Source: CAD feature listing. Evaluate the final solid. Frame: model axes, mm. Face numbers are marked on the shaded views. A direction names the side the tool comes from. Give positions to 0.01 mm unless a question says otherwise; leave off trailing zeros. Order: outer loops, then holes, each group sorted by start corner. A loop starts at its lowest first (then second) coordinate and runs counter-clockwise, first axis right, second up. Notation, with made-up numbers: M 76.25,8 L 133.25,8 A22 cw 133.25,38 Z; hole C 1,40.5 d8. An arc over 180 degrees is marked long. Answer as a JSON object with one key per item and string values. Group by question number.
1. Pin query (flat end, axial travel): P1, Ø6, axis at x = 14, y = 11.5, coming from the +Z side (3 decimals); P2, Ø1.3, axis at x = -0.5, z = -34, coming from the -Y side; P3, Ø1.3, axis at x = -0.5, y = 1.5, coming from the +Z side (3 decimals); P4, Ø4.5, axis at y = 4.15, z = -61.79, coming from the -X side (1 decimal). Return the tip coordinate at first contact, or that it passes through.
2. Set-up query: the marked faces 4 and 5. Return all of +Z, -Z, +X, -X, +Y, -Y with unobstructed straight access to the full face (end or side cutting, diameter ignored); none if empty.
3. Material intervals for L1, parallel to X at y = 5, z = -16.5 (1 decimal); L2, parallel to Y at x = 8.5, z = -21.5 (1 decimal); L3, parallel to Y at x = 16.25, z = -6, sorted ascending. Write a range as [from, to].
4. Pull-direction query (X, two-part tool) for the marked faces 1, 2 and 3; classes: +X half, -X half, draft (parallel to the pull), parting line (faces both ways), or undercut.
5. Section query B-B (z = -60.5). Output: boundary loops of the cut face in (x, y) (1 decimal), plus the area to 3 significant figures.
6. Section query D-D (z = -19). Output: boundary loops of the cut face in (x, y) (1 decimal), plus the area to 3 significant figures.
7. Section query C-C (y = 5). Count the separate pieces of the cut face and the enclosed holes in it, plus the area to 3 significant figures.
8. Section query A-A (y = 10.75). Output: boundary loops of the cut face in (x, z) (1 decimal), plus the area to 3 significant figures.
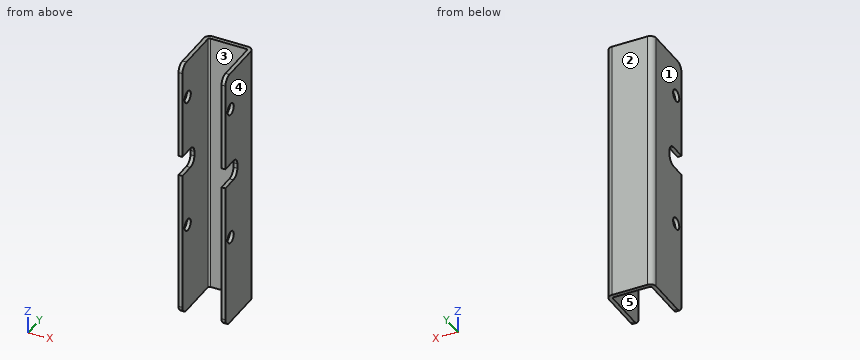
from build123d import *

# Parameters (mm, degrees)
BASE_FLANGE1_DEPTH           = 1.5875
EDGE_FLANGE1_STRIP_W         = 7.8232
EDGE_FLANGE1_STRIP_H         = 1.5875
EDGE_FLANGE1_STRIP_CUT_DEPTH = 107.95
EDGE_FLANGE1_DEPTH           = 107.95
EDGE_FLANGE2_STRIP_W         = 7.8232
EDGE_FLANGE2_STRIP_H         = 1.5875
EDGE_FLANGE2_STRIP_CUT_DEPTH = 107.95
EDGE_FLANGE2_DEPTH           = 107.95
HOLE1_START                  = -1.5875
HOLE1_OUTLINE_R              = 2.413
HOLE1_DEPTH                  = 19.05
CUT_EXTRUDE1_DEPTH           = 103.402979235
CUT_EXTRUDE1_DEPTH_BACK      = 103.402979235
SKETCH27_W                   = 8.255
SKETCH27_H                   = 9.364783331
FILLET1_R                    = 3.175


# Read off the part's stored shape, not the designer's step: Hole1
# Sheet-metal steps are written as plain solids
with BuildPart() as part:
    # Sketch1 → Base-Flange1 (new body)
    with BuildSketch(Plane(origin=(0, 0, 0), x_dir=(0, 0, -1), z_dir=(1, 0, 0))):
        Polygon((0, 0), (88.9, 0), (98.425, 0), (98.425, 22.225), (88.9, 22.225), (0, 22.225), (-9.525, 22.225), (-9.525, 0), align=None)
    extrude(amount=-BASE_FLANGE1_DEPTH)

    # Edge-Flange1 strip (across the edge) → Edge-Flange1 strip cut (cut)
    with BuildSketch(Plane(origin=(0, 22.225, -98.425), x_dir=(0, -1, 0), z_dir=(0, 0, 1))):
        with Locations((-1.5875, -0.79375)):
            Rectangle(EDGE_FLANGE1_STRIP_W, EDGE_FLANGE1_STRIP_H)
    extrude(amount=EDGE_FLANGE1_STRIP_CUT_DEPTH, mode=Mode.SUBTRACT)

    # Edge-Flange1 section (across the edge) → Edge-Flange1 (add)
    with BuildSketch(Plane(origin=(0, 22.225, -98.425), x_dir=(0, -1, 0), z_dir=(0, 0, 1))):
        with BuildLine():
            Line((0, 0.7366), (0, 17.4625))
            Line((0, 17.4625), (1.5875, 17.4625))
            Line((1.5875, 17.4625), (1.5875, 0.7366))
            ThreePointArc((1.5875, 0.7366), (1.803245145, 0.215745145), (2.3241, 0))
            Line((2.3241, 0), (2.3241, -1.5875))
            ThreePointArc((2.3241, -1.5875), (0.68071313, -0.90678687), (0, 0.7366))
        make_face()
    extrude(amount=EDGE_FLANGE1_DEPTH)

    # Edge-Flange2 strip (across the edge) → Edge-Flange2 strip cut (cut)
    with BuildSketch(Plane(origin=(17.4625, 20.6375, -98.425), x_dir=(-1, 0, 0), z_dir=(0, 0, 1))):
        with Locations((-1.5875, -0.79375)):
            Rectangle(EDGE_FLANGE2_STRIP_W, EDGE_FLANGE2_STRIP_H)
    extrude(amount=EDGE_FLANGE2_STRIP_CUT_DEPTH, mode=Mode.SUBTRACT)

    # Edge-Flange2 section (across the edge) → Edge-Flange2 (add)
    with BuildSketch(Plane(origin=(17.4625, 20.6375, -98.425), x_dir=(-1, 0, 0), z_dir=(0, 0, 1))):
        with BuildLine():
            Line((0, 0.7366), (0, 20.6375))
            Line((0, 20.6375), (1.5875, 20.6375))
            Line((1.5875, 20.6375), (1.5875, 0.7366))
            ThreePointArc((1.5875, 0.7366), (1.803245145, 0.215745145), (2.3241, 0))
            Line((2.3241, 0), (2.3241, -1.5875))
            ThreePointArc((2.3241, -1.5875), (0.68071313, -0.90678687), (0, 0.7366))
        make_face()
    extrude(amount=EDGE_FLANGE2_DEPTH)

    # Hole1 outline → Hole1 (cut)
    with BuildSketch(Plane.YZ.offset(HOLE1_START)):
        with Locations((4.148353843, -61.790618702)):
            Circle(HOLE1_OUTLINE_R)
        with Locations((4.148353843, -6.164618702)):
            Circle(HOLE1_OUTLINE_R)
    extrude(amount=HOLE1_DEPTH, mode=Mode.SUBTRACT)

    # Sketch27 → Cut-Extrude1 (cut, two sides: drawn at the far end of the back side and taken through both)
    with BuildSketch(Plane(origin=(0, 0, 0), x_dir=(0, 0, -1), z_dir=(1, 0, 0)).offset(-CUT_EXTRUDE1_DEPTH_BACK)):
        with Locations((33.9725, 4.682391665)):
            Rectangle(SKETCH27_W, SKETCH27_H)
    extrude(amount=CUT_EXTRUDE1_DEPTH + CUT_EXTRUDE1_DEPTH_BACK, mode=Mode.SUBTRACT)

    # Fillet1
    fillet1_edges = [part.edges().sort_by_distance(p)[0] for p in [
        (-0.79375, 9.364783331, -29.845),
        (-0.79375, 9.364783331, -38.1),
        (16.66875, 9.364783331, -29.845),
        (16.66875, 9.364783331, -38.1),
        (-0.79375, 0, 9.525),
        (-0.79375, 0, -98.425),
        (16.66875, 0, -98.425),
        (16.66875, 0, 9.525),
    ]]
    fillet(fillet1_edges, radius=FILLET1_R)


solid = part.part
Answer sheet:
{
 "1": {"P1": "z = 9.525", "P2": "y = 9.36", "P3": "z = 9.355", "P4": "through"},
 "2": {"face 4": "+Z, -Z, +X, +Y, -Y", "face 5": "+Z, -Z, -Y"},
 "3": {"L1": "[-1.6, 0], [15.9, 17.5]", "L2": "[20.6, 22.2]", "L3": "[0, 1.74], [6.56, 21.94]"},
 "4": {"face 1": "-X half", "face 2": "draft", "face 3": "undercut"},
 "5": {"outline": "M -1.6,0 L 0,0 L 0,2.1 L -1.6,2.1 Z; M -1.6,6.2 L 0,6.2 L 0,19.9 A0.7 cw 0.7,20.6 L 15.1,20.6 A0.7 cw 15.9,19.9 L 15.9,6.2 L 17.5,6.2 L 17.5,19.9 A2.3 ccw 15.1,22.2 L 0.7,22.2 A2.3 ccw -1.6,19.9 Z; M 15.9,0 L 17.5,0 L 17.5,2.1 L 15.9,2.1 Z", "area": "80.7 mm^2"},
 "6": {"outline": "M -1.6,0 L 0,0 L 0,19.9 A0.7 cw 0.7,20.6 L 15.1,20.6 A0.7 cw 15.9,19.9 L 15.9,0 L 17.5,0 L 17.5,19.9 A2.3 ccw 15.1,22.2 L 0.7,22.2 A2.3 ccw -1.6,19.9 Z", "area": "93.7 mm^2"},
 "7": {"separate pieces": "8", "enclosed holes": "0", "area": "288 mm^2"},
 "8": {"outline": "M -1.6,-98.4 L 0,-98.4 L 0,9.5 L -1.6,9.5 Z; M 15.9,-98.4 L 17.5,-98.4 L 17.5,9.5 L 15.9,9.5 Z", "area": "343 mm^2"}
}
